from build123d import *

# Parameters (mm, degrees)
F0_W     = 38.1
F0_H     = 38.1
F1_DEPTH = 38.1
F3_DEPTH = 38.1


with BuildPart() as f1:
    # F0 (on Top) → F1 (new body)
    with BuildSketch(Plane.XY):
        with Locations((2.80316, -7.937101)):
            Rectangle(F0_W, F0_H)
    extrude(amount=F1_DEPTH)

    # F2 (on face) → F3 (join)
    with BuildSketch(Plane.YZ.offset(21.85316)):
        Polygon((11.112899, 0), (11.112899, 25.4), (-14.287101, 0), align=None)
    extrude(amount=F3_DEPTH)


solid = f1.part
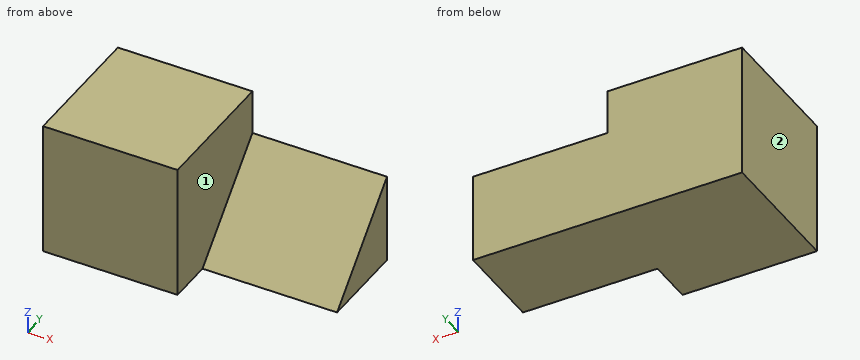
Build history of the part. All positions in model axes, mm. Face numbers are marked on the shaded views. A direction names the side the tool comes from. Round coordinates to 2 decimals unless told otherwise and drop trailing zeros. Write each loop counter-clockwise with the first axis right and the second up, starting at its lowest first coordinate (ties: lowest second). Pieces come first, ordered by that corner, then holes. Notation, with made-up numbers: M -6,56 L 20,56 A15 cw 20,77 Z; hole C 76,47.5 d2. An arc over 180 degrees is marked long. Answer as a JSON object with one key per item and string values. Group by question number.
(1) Drill centre lines: L1, parallel to X at y = -21, z = 20.5; L2, parallel to Y at x = 55, z = 12; L3, parallel to Z at x = 56.5, y = 9. Where is each one in solid material? Low to high.
(2) Cut at D-D (z = 28). Give the cut face in (x, y).
(3) Cut at C-C (x = 42.5). Give the cut face in (y, z).
(4) Flat gauge pin, fed straight in: pin 1 (3 mm diameter, centred on y = -12, z = 14, fed in from +X). Where does the tip first touch, or does it go through?
(5) Cut at B-B (y = 6.5). Give the cut face in (x, z), and give its area (3 significant figures).
(6) Which spindle directions (+Z, -Z, +X, -X, +Y, -Y) get a long thin tool onto all of the face, cutting with end or side? Do the marked faces 1 and 2. Say none if no direction does.
(7) Cut at A-A (z = 23). Give the cut face in (x, y), and give its area (3 significant figures).
Responses:
{
 "1": {"L1": "x = -16.25 to 21.85", "L2": "y = -2.29 to 11.11", "L3": "z = 0 to 23.29"},
 "2": {"outline": "M -16.25,-26.99 L 21.85,-26.99 L 21.85,11.11 L -16.25,11.11 Z"},
 "3": {"outline": "M -14.29,0 L 11.11,0 L 11.11,25.4 Z"},
 "4": {"pin 1": "stops at x = 21.85"},
 "5": {"outline": "M -16.25,0 L 59.95,0 L 59.95,20.79 L 21.85,20.79 L 21.85,38.1 L -16.25,38.1 Z", "area": "2,240 mm2"},
 "6": {"face 1": "+Z, +X, -Y", "face 2": "+Z, -Z, -X, +Y, -Y"},
 "7": {"outline": "M -16.25,-26.99 L 21.85,-26.99 L 21.85,8.71 L 59.95,8.71 L 59.95,11.11 L -16.25,11.11 Z", "area": "1,540 mm2"}
}
